Check sheet for the modelled part. Datum: model origin and axes. Units: mm. Face numbers are marked on the shaded views. A direction names the side the tool comes from. Coordinates: 2 decimals unless noted, no trailing zeros. Order: outer loops, then holes, each group sorted by start corner. A loop starts at its lowest first (then second) coordinate and runs counter-clockwise, first axis right, second up.
1. Cross-section at A-A (x = 100). Enter the section's corners in (y, z).
2. Thickness scan on line 1 (Z direction, x = 93.5, y = -11); line 2 (X direction, y = -17, z = 15); line 3 (Z direction, x = -23, y = 36). Record the ranges inside material, lowest first.
3. Set-up check for the marked faces 1, 2 and 3: record each of +Z, -Z, +X, -X, +Y, -Y from which the full face is reachable in a straight line by a thin tool's end or side.
4. Cross-section at D-D (y = 22.5). Enter the section's corners in (x, z), then the cut area to 3 significant figures.
5. Gauge pin test, flat ends, axial feed: pin 1 Ø3.5 at (y, z) = (5.5, -2) entering from +X; pin 2 Ø12 at (y, z) = (-8.5, -1.5) entering from -X; pin 3 Ø8 at (x, z) = (81.5, -2.5) entering from +Y; pin 4 Ø10 at (x, y) = (0, -13.98) entering from +Z. Record the tip position at first contact, or that the pin passes through.
6. Cross-section at C-C (z = 0.5). Enter the section's corners in (x, y).
7. Draft check along Z on the marked faces 4, 5 and 6. Enter one of: released by +Z, released by -Z, zero draft, split by the parting line, or undercut.
8. Cross-section at B-B (x = 34). Enter the section's corners in (y, z).
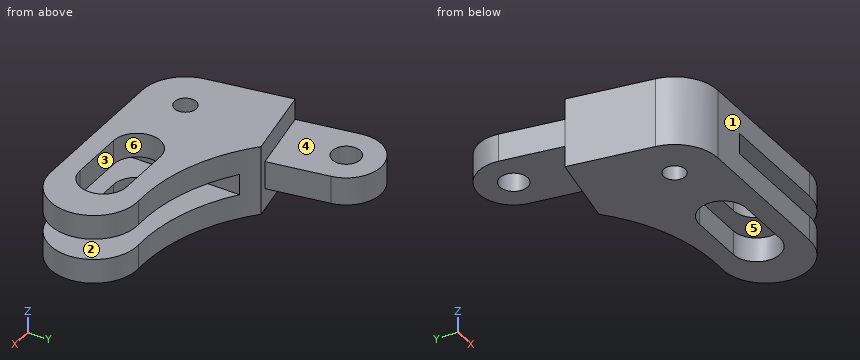
```python
from build123d import *

# Parameters (mm, degrees)
SKETCH1_R                = 6.25
BOSS_EXTRUDE1_DEPTH      = 20
CUT_EXTRUDE2_DEPTH       = 6
BOSS_EXTRUDE2_DEPTH      = 8
BOSS_EXTRUDE2_DEPTH_BACK = 8
SKETCH8_R                = 8
CUT_EXTRUDE3_DEPTH       = 143.929611875


with BuildPart() as part:
    # Sketch1 → Boss-Extrude1 (new, symmetric)
    with BuildSketch(Plane.XY):
        with BuildLine():
            Line((0, -38.979129488), (85, -38.979129488))
            ThreePointArc((85, -38.979129488), (109.991458118, -13.325660942), (83.693509457, 10.986708821))
            ThreePointArc((83.693509457, 10.986708821), (44.909838533, 16.648787206), (11.281411091, 36.782369345))
            Line((11.281411091, 36.782369345), (-33.022622734, 28.898678149))
            Line((-33.022622734, 28.898678149), (-24.613352125, -18.35895793))
            ThreePointArc((-24.613352125, -18.35895793), (-16.054661145, -33.142841433), (0, -38.979129488))
        make_face()
        with Locations((0, -13.979129488)):
            Circle(SKETCH1_R, mode=Mode.SUBTRACT)
        with BuildLine():
            Line((45, -0.479129488), (76.239117398, -0.479129488))
            ThreePointArc((76.239117398, -0.479129488), (89.739117398, -13.979129488), (76.239117398, -27.479129488))
            Line((76.239117398, -27.479129488), (45, -27.479129488))
            ThreePointArc((45, -27.479129488), (31.5, -13.979129488), (45, -0.479129488))
        make_face(mode=Mode.SUBTRACT)
    extrude(amount=BOSS_EXTRUDE1_DEPTH, both=True)

    # Sketch5 → Cut-Extrude2 (cut, symmetric)
    with BuildSketch(Plane.XY):
        with BuildLine():
            Line((20, 29.723334557), (20, -38.979129488))
            Line((20, -38.979129488), (85, -38.979129488))
            ThreePointArc((85, -38.979129488), (109.991458118, -13.325660942), (83.693509457, 10.986708821))
            ThreePointArc((83.693509457, 10.986708821), (50.246422532, 14.914833293), (20, 29.723334557))
        make_face()
    extrude(amount=CUT_EXTRUDE2_DEPTH, both=True, mode=Mode.SUBTRACT)

    # Sketch7 → Boss-Extrude2 (add, two sides: drawn at the far end of the back side and taken through both)
    with BuildSketch(Plane.XY.offset(-BOSS_EXTRUDE2_DEPTH_BACK)):
        with BuildLine():
            Line((-33.022622734, 28.898678149), (6.358740666, 35.906403657))
            Line((6.358740666, 35.906403657), (0.226980847, 70.365096632))
            ThreePointArc((0.226980847, 70.365096632), (0.458819494, 68.619978601), (0.536299147, 66.861233878))
            ThreePointArc((0.536299147, 66.861233878), (-17.70495613, 46.93871353), (-39.154382553, 63.357371124))
            Line((-39.154382553, 63.357371124), (-33.022622734, 28.898678149))
        make_face()
        with BuildLine():
            ThreePointArc((0.536299147, 66.861233878), (0.458819494, 68.619978601), (0.226980847, 70.365096632))
            Line((0.226980847, 70.365096632), (-39.154382553, 63.357371124))
            ThreePointArc((-39.154382553, 63.357371124), (-17.70495613, 46.93871353), (0.536299147, 66.861233878))
        make_face()
        with BuildLine():
            Line((-39.154382553, 63.357371124), (0.226980847, 70.365096632))
            ThreePointArc((0.226980847, 70.365096632), (-22.967563607, 86.551915578), (-39.154382553, 63.357371124))
        make_face()
    extrude(amount=BOSS_EXTRUDE2_DEPTH + BOSS_EXTRUDE2_DEPTH_BACK)

    # Sketch8 → Cut-Extrude3 (cut, through all)
    with BuildSketch(Plane.XY.offset(8)):
        with Locations((-19.463700853, 66.861233878)):
            Circle(SKETCH8_R)
    extrude(amount=-CUT_EXTRUDE3_DEPTH, mode=Mode.SUBTRACT)


solid = part.part
```
Data:
1. outline: (-33.98, -20) - (6.02, -20) - (6.02, -6) - (-33.98, -6) - close; (-33.98, 6) - (6.02, 6) - (6.02, 20) - (-33.98, 20) - close
2. line 1: z = -20 to -6, 6 to 20
2. line 2: x = -24.86 to -5.47, 5.47 to 31.84, 89.4 to 109.82
2. line 3: z = -8 to 8
3. face 1: +Z, -Z, +X, -X, -Y
3. face 2: +X, +Y, -Y
3. face 3: +Z, -Z
4. outline: (-31.88, -20) - (31.62, -20) - (31.62, -6) - (20, -6) - (20, 6) - (31.62, 6) - (31.62, 20) - (-31.88, 20) - close
4. area: 2,400 mm2
5. pin 1: stops at x = 20
5. pin 2: stops at x = -27.44
5. pin 3: stops at y = 10.97
5. pin 4: passes through
6. outline: (-39.15, 63.36) - (-24.61, -18.36) arc R25 ccw to (0, -38.98) - (20, -38.98) - (20, 29.72) arc R100 cw to (11.28, 36.78) - (6.36, 35.91) - (0.23, 70.37) arc R20 ccw to start; hole circle Ø16 at (-19.46, 66.86); hole circle Ø12.5 at (0, -13.98)
7. face 4: released by +Z
7. face 5: undercut
7. face 6: zero draft
8. outline: (-38.98, -20) - (-21.81, -20) - (-21.81, -6) - (-38.98, -6) - close; (-38.98, 6) - (-21.81, 6) - (-21.81, 20) - (-38.98, 20) - close; (-6.15, -20) - (21.28, -20) - (21.28, -6) - (-6.15, -6) - close; (-6.15, 6) - (21.28, 6) - (21.28, 20) - (-6.15, 20) - close
